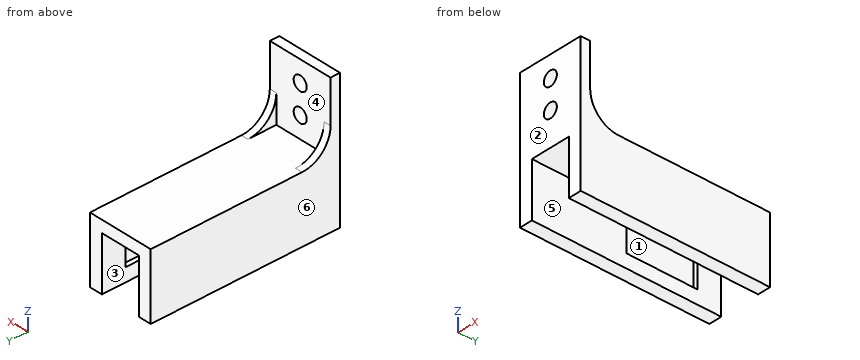
```python
from build123d import *

# Parameters (mm, degrees)
SKETCH1_W           = 14
SKETCH1_H           = 40
BOSS_EXTRUDE1_DEPTH = 14
SKETCH2_W           = 10.4
SKETCH2_H           = 8.65
SKETCH2_W_2         = 8.5
SKETCH2_H_2         = 2.85
CUT_EXTRUDE1_DEPTH  = 35
SKETCH3_W           = 14
SKETCH3_H           = 15
SKETCH3_R           = 1.5
BOSS_EXTRUDE2_DEPTH = 2
BOSS_EXTRUDE3_DEPTH = 1.5
SKETCH5_W           = 8.5
SKETCH5_H           = 11.5
CUT_EXTRUDE2_DEPTH  = 46.98912915
SKETCH7_W           = 0.95
SKETCH7_H           = 8.65
BOSS_EXTRUDE4_DEPTH = 20


with BuildPart() as part:
    # Sketch1 → Boss-Extrude1 (new body)
    with BuildSketch(Plane.XY):
        Rectangle(SKETCH1_W, SKETCH1_H)
    extrude(amount=BOSS_EXTRUDE1_DEPTH)

    # Sketch2 → Cut-Extrude1 (cut)
    with BuildSketch(Plane.XZ.offset(20)):
        with Locations((0, 7.175)):
            Rectangle(SKETCH2_W, SKETCH2_H)
        with Locations((0, 1.425)):
            Rectangle(SKETCH2_W_2, SKETCH2_H_2)
    extrude(amount=-CUT_EXTRUDE1_DEPTH, mode=Mode.SUBTRACT)

    # Sketch3 → Boss-Extrude2 (add)
    with BuildSketch(Plane.XZ.offset(20)):
        with Locations((0, 21.5)):
            Rectangle(SKETCH3_W, SKETCH3_H)
        with Locations((0, 18.5)):
            Circle(SKETCH3_R, mode=Mode.SUBTRACT)
        with Locations((0, 24.5)):
            Circle(SKETCH3_R, mode=Mode.SUBTRACT)
    extrude(amount=-BOSS_EXTRUDE2_DEPTH)

    # Sketch4 → Boss-Extrude3 (add)
    with BuildSketch(Plane.ZY.offset(7)):
        with BuildLine():
            Line((14, -12), (14, -18))
            Line((14, -18), (20, -18))
            ThreePointArc((20, -18), (15.757359313, -16.242640687), (14, -12))
        make_face()
    boss_extrude3 = extrude(amount=-BOSS_EXTRUDE3_DEPTH)

    # Mirror1: Boss-Extrude3 across plane
    add(boss_extrude3.mirror(Plane(origin=(0, 0, 0), x_dir=(0, 0, 1), z_dir=(1, 0, 0))))

    # Sketch5 → Cut-Extrude2 (cut, through all)
    with BuildSketch(Plane.XZ.offset(-15)):
        with Locations((0, 5.75)):
            Rectangle(SKETCH5_W, SKETCH5_H)
    extrude(amount=-CUT_EXTRUDE2_DEPTH, mode=Mode.SUBTRACT)

    # Sketch7 → Boss-Extrude4 (add)
    with BuildSketch(Plane.XZ.offset(20)):
        with Locations((4.725, 7.175)):
            Rectangle(SKETCH7_W, SKETCH7_H)
        with Locations((-4.725, 7.175)):
            Rectangle(SKETCH7_W, SKETCH7_H)
    extrude(amount=-BOSS_EXTRUDE4_DEPTH)


solid = part.part
```
Could you check a few things on this model? Use its own coordinates, in mm. Face numbers are marked on the shaded views. A direction names the side the tool comes from. Round coordinates to 2 decimals unless told otherwise and drop trailing zeros. Loops run counter-clockwise (first coordinate to the right, second up) from the corner with the lowest first, then second, coordinate; pieces in that order, holes last.
Q1. Thinking about a two-plate mould opening in Y: for the marked faces 1, 2 and 3, which applies, pulls with the +Y half, pulls with the -Y half, needs draft (parallel to the pull), parting line crosses it, or undercut?
Q2. On a 3-axis mill with a long thin cutter (end or side, diameter ignored), from which of +Z, -Z, +X, -X, +Y, -Y can I reach the whole of each face in a straight line? I mean the marked faces 4, 5 and 6. Say none if no direction works.
Q3. I want a section at B-B (x = 0). Write out the boundary of the cut face in (y, z), and give its area (3 significant figures).
Q4. Please list where these lines run through material, in increasing order: L1, parallel to Z at x = 0, y = -18.35; L2, parallel to X at y = 10, z = 2.75; L3, parallel to Y at x = 4.5, z = 11.
Q5. For P1, Ø5, axis at x = 0, z = 24.5, coming from the -Y side; P2, Ø1, axis at x = -5.5, y = 3.5, coming from the +Z side; P3, Ø4, axis at x = 3, z = 23.5, coming from the +Y side; P4, Ø2, axis at x = 2.5, y = -15, coming from the -Z side, each with a flat end and sliding along its axis, tell me the tip position at first contact or that it passes through.
Q6. I want a section at D-D (x = -3.5). Write out the boundary of the cut face in (y, z), and give its area (3 significant figures).
Q7. I want a section at A-A (z = 24.5). Write out the boundary of the cut face in (x, y).
Q8. I want a section at C-C (y = 14). Write out the boundary of the cut face in (x, z), and give its area (3 significant figures).
Answer below:
1. face 1: undercut
1. face 2: pulls with the -Y half
1. face 3: needs draft
2. face 4: +Z, +Y
2. face 5: -Z, +Y, -Y
2. face 6: +Z, -Z, -X, +Y, -Y
3. outline: (-20, 11.5) - (20, 11.5) - (20, 14) - (-18, 14) - (-18, 17) - (-20, 17) - close; (-20, 20) - (-18, 20) - (-18, 23) - (-20, 23) - close; (-20, 26) - (-18, 26) - (-18, 29) - (-20, 29) - close
3. area: 118 mm2
4. L1: z = 11.5 to 17, 20 to 23, 26 to 29
4. L2: x = -7 to -4.25, 4.25 to 7
4. L3: y = -20 to 0, 15 to 20
5. P1: stops at y = -20
5. P2: stops at z = 14
5. P3: stops at y = -18
5. P4: stops at z = 11.5
6. outline: (-20, 11.5) - (20, 11.5) - (20, 14) - (-18, 14) - (-18, 29) - (-20, 29) - close
6. area: 130 mm2
7. outline: (-7, -20) - (-1.5, -20) - (-1.5, -18) - (-7, -18) - close; (1.5, -20) - (7, -20) - (7, -18) - (1.5, -18) - close
8. outline: (-7, 0) - (-4.25, 0) - (-4.25, 2.85) - (-5.2, 2.85) - (-5.2, 11.5) - (5.2, 11.5) - (5.2, 2.85) - (4.25, 2.85) - (4.25, 0) - (7, 0) - (7, 14) - (-7, 14) - close
8. area: 81.8 mm2
